For this review, take the finished solid that the model builds, in its own axes (mm). Face numbers are marked on the shaded views. A direction names the side the tool comes from. Coordinates: 2 decimals unless noted, no trailing zeros. Write each loop counter-clockwise with the first axis right and the second up, starting at its lowest first coordinate (ties: lowest second). Pieces come first, ordered by that corner, then holes. Notation, with made-up numbers: (27, -28.75) - (58, -28.75) arc R11 cw to (58, -20.75) - close; hole circle Ø6 at (-1.5, 55). An arc over 180 degrees is marked (long way). Write each question's results on one line, items separated by ' | '.
from build123d import *

# Parameters (mm, degrees)
F0_W     = 76.2
F0_H     = 50.8
F1_DEPTH = 12.7
F3_DEPTH = 12.7
F2_W     = 1.27
F2_H     = 50.8
F4_DEPTH = 5.08
F6_DEPTH = 50.8
F7_R     = 4.7625
F8_DEPTH = 12.7


with BuildPart() as f1:
    # F0 (on Front) → F1 (new body)
    with BuildSketch(Plane.XZ):
        Rectangle(F0_W, F0_H)
    extrude(amount=F1_DEPTH)

    # F2 (on face) → F3 (cut)
    with BuildSketch(Plane.XZ.offset(12.7)):
        with BuildLine():
            Line((-6.35, -10.994409386), (-6.35, 10.994409386))
            ThreePointArc((-6.35, 10.994409386), (-12.6964379944, 0), (-6.35, -10.994409386))
        make_face()
        with BuildLine():
            ThreePointArc((6.35, 10.994409386), (0, 12.6964379944), (-6.35, 10.994409386))
            Line((-6.35, 10.994409386), (-6.35, -10.994409386))
            ThreePointArc((-6.35, -10.994409386), (0, -12.6964379944), (6.35, -10.994409386))
            Line((6.35, -10.994409386), (6.35, 10.994409386))
        make_face()
        with BuildLine():
            ThreePointArc((12.6964379944, 0), (10.99595196, 6.3473284334), (6.35, 10.994409386))
            Line((6.35, 10.994409386), (6.35, -10.994409386))
            ThreePointArc((6.35, -10.994409386), (10.99595196, -6.3473284334), (12.6964379944, 0))
        make_face()
    extrude(amount=-F3_DEPTH, mode=Mode.SUBTRACT)

    # F2 (on face) → F4 (cut)
    with BuildSketch(Plane.XZ.offset(12.7)):
        with Locations((-34.925, 0)):
            Rectangle(F2_W, F2_H)
        with BuildLine():
            ThreePointArc((6.35, -10.994409386), (10.99595196, -6.3473284334), (12.6964379944, 0))
            ThreePointArc((12.6964379944, 0), (10.99595196, 6.3473284334), (6.35, 10.994409386))
            Line((6.35, 10.994409386), (6.35, -10.994409386))
        make_face()
        with BuildLine():
            Line((6.35, -10.994409386), (6.35, 10.994409386))
            ThreePointArc((6.35, 10.994409386), (0, 12.6964379944), (-6.35, 10.994409386))
            Line((-6.35, 10.994409386), (-6.35, -10.994409386))
            ThreePointArc((-6.35, -10.994409386), (0, -12.6964379944), (6.35, -10.994409386))
        make_face()
        with BuildLine():
            ThreePointArc((-6.35, 10.994409386), (0, 12.6964379944), (6.35, 10.994409386))
            Line((6.35, 10.994409386), (6.35, 25.4))
            Line((6.35, 25.4), (-6.35, 25.4))
            Line((-6.35, 25.4), (-6.35, 10.994409386))
        make_face()
        with BuildLine():
            Line((6.35, -25.4), (6.35, -10.994409386))
            ThreePointArc((6.35, -10.994409386), (0, -12.6964379944), (-6.35, -10.994409386))
            Line((-6.35, -10.994409386), (-6.35, -25.4))
            Line((-6.35, -25.4), (6.35, -25.4))
        make_face()
        with BuildLine():
            Line((-6.35, -10.994409386), (-6.35, 10.994409386))
            ThreePointArc((-6.35, 10.994409386), (-12.6964379944, 0), (-6.35, -10.994409386))
        make_face()
    extrude(amount=-F4_DEPTH, mode=Mode.SUBTRACT)

    # F5 (on face) → F6 (cut)
    with BuildSketch(Plane(origin=(0, 0, -25.4), x_dir=(1, 0, 0), z_dir=(0, 0, -1))):
        Polygon((25.7032178342, 12.7), (19.0220633893, 12.7), (16.0891240218, 7.62), (28.6361572017, 7.62), align=None)
    extrude(amount=-F6_DEPTH, mode=Mode.SUBTRACT)

    # F7 (on face) → F8 (join)
    with BuildSketch(Plane.YZ.offset(38.1)):
        with Locations((-6.35, 0)):
            Circle(F7_R)
    extrude(amount=F8_DEPTH)


solid = f1.part
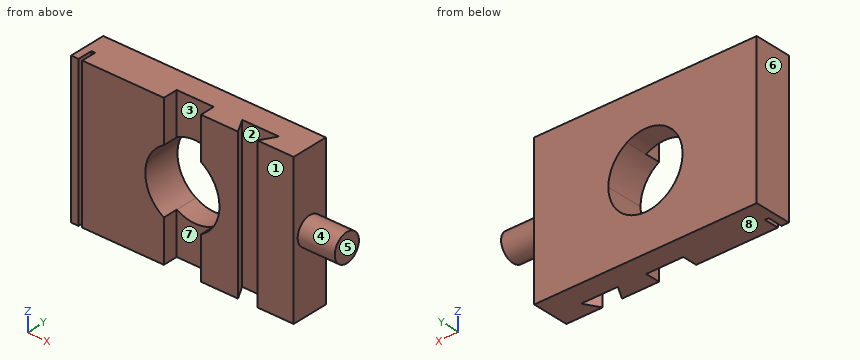
Q1. Wall thickness on line 1 along X through (y, z) = (-10.5, 16.5); line 2 along X through (y, z) = (-10, -6.5); line 3 along X through (y, z) = (-4, -19): over which ranges is each line inside the solid? List them lowest first. Write a range as from..to.
Results found:
line 1: -38.1..-35.56, -34.29..-6.35, 6.35..17.75, 26.97..38.1 | line 2: -38.1..-35.56, -34.29..-10.91, 10.91..17.46, 27.26..38.1 | line 3: -38.1..38.1
Q2. Mouldability with a two-part tool opening along X and no side actions: class the marked faces 5, 6, 7 and 8 as pulls with the +X half, pulls with the -X half, needs draft (parallel to the pull), parting line crosses it, or undercut.
Results found:
face 5: pulls with the +X half | face 6: pulls with the -X half | face 7: undercut | face 8: needs draft
Q3. For the marked faces 1, 2, 3 and 4, list the 3-axis set-ups (+Z, -Z, +X, -X, +Y, -Y) from which the entire face can be reached by the end or side of a thin tool; tool diameter is ignored.
Results found:
face 1: +Z, -Z, +X, -X, -Y | face 2: +Z, -Z | face 3: +Z, -Z, -Y | face 4: +X
Q4. Take a section at C-C on z = -2.5. State the section outline as (x, y) points, plus the area to 3 significant figures.
Results found:
outline: (-38.1, -12.7) - (-35.56, -12.7) - (-35.56, -7.62) - (-34.29, -7.62) - (-34.29, -12.7) - (-12.45, -12.7) - (-12.45, 0) - (-38.1, 0) - close; (12.45, -12.7) - (19.02, -12.7) - (16.09, -7.62) - (28.64, -7.62) - (25.7, -12.7) - (38.1, -12.7) - (38.1, -10.4) - (50.8, -10.4) - (50.8, -2.3) - (38.1, -2.3) - (38.1, 0) - (12.45, 0) - close | area: 699 mm2
Q5. Take a section at A-A on y = -6.35. State the section outline as (x, z) points, plus the area to 3 significant figures.
Results found:
outline: (-38.1, -25.4) - (38.1, -25.4) - (38.1, -4.76) - (50.8, -4.76) - (50.8, 4.76) - (38.1, 4.76) - (38.1, 25.4) - (-38.1, 25.4) - close; hole circle Ø25.39 at (0, 0) | area: 3,490 mm2
Q6. For pin 1 (6.5 mm diameter, centred on x = -2.5, z = -18.5, fed in from -Y); pin 2 (5.5 mm diameter, centred on y = -9, z = -17.5, fed in from +X), all flat-tipped, find the tip position at first contact; note any pin that passes through.
Results found:
pin 1: y = -7.62 | pin 2: x = 38.1
Q7. Take a section at B-B on x = -8.5. State the section outline as (y, z) points.
Results found:
outline: (-12.7, -25.4) - (0, -25.4) - (0, -9.43) - (-12.7, -9.43) - close; (-12.7, 9.43) - (0, 9.43) - (0, 25.4) - (-12.7, 25.4) - close
Q8. Take a section at D-D on z = 21. State the section outline as (x, y) points, plus the area to 3 significant figures.
Results found:
outline: (-38.1, -12.7) - (-35.56, -12.7) - (-35.56, -7.62) - (-34.29, -7.62) - (-34.29, -12.7) - (-6.35, -12.7) - (-6.35, -7.62) - (6.35, -7.62) - (6.35, -12.7) - (19.02, -12.7) - (16.09, -7.62) - (28.64, -7.62) - (25.7, -12.7) - (38.1, -12.7) - (38.1, 0) - (-38.1, 0) - close | area: 848 mm2
